Input: part model. Units: mm. Frame: model coordinates. Face numbers are marked on the shaded views. A direction names the side the tool comes from. Coordinates: 2 decimals unless noted, no trailing zeros. Write each loop counter-clockwise with the first axis right and the second up, starting at its lowest first coordinate (ties: lowest second). Pieces come first, ordered by that corner, then holes. Notation, with made-up numbers: (-20.5, 35) -> (-8.5, 35) arc R16 cw to (-8.5, 51) -> close; hole circle Ø11 at (-17.75, 41). An arc over 180 degrees is marked (long way). One line per question, with ' | ' between items. Start each with the question number.
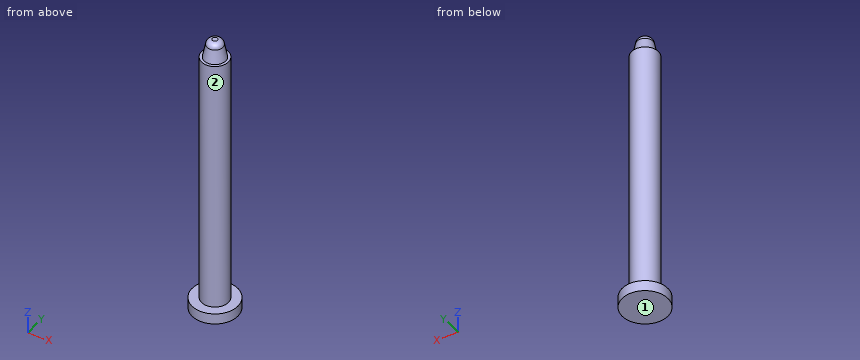
```python
from build123d import *

# Parameters (mm, degrees)
F0_R     = 8.5
F1_DEPTH = 4
F2_R     = 5
F3_DEPTH = 100


with BuildPart() as f1:
    # F0 (on Top) → F1 (new body)
    with BuildSketch(Plane.XY):
        Circle(F0_R)
    extrude(amount=F1_DEPTH)

    # F2 (on Top) → F3 (join)
    with BuildSketch(Plane.XY):
        Circle(F2_R)
    extrude(amount=F3_DEPTH)

    # F4 (on Right) → F5 (revolve)
    with BuildSketch(Plane.YZ):
        Polygon((3, 105), (0, 105), (0, 100), (4, 100), align=None)
    revolve(axis=Axis((0, 0, 102.5), (0, 0, -1)))

    # F6 (on Right) → F7 (revolve)
    with BuildSketch(Plane.YZ):
        with BuildLine():
            Line((1, 107), (0, 107))
            Line((0, 107), (0, 105))
            Line((0, 105), (3, 105))
            ThreePointArc((3, 105), (2.414214, 106.414214), (1, 107))
        make_face()
    revolve(axis=Axis((0, 0, 106), (0, 0, -1)))


solid = f1.part
```
1) Section B-B, the plane y = 7.5. Return loops of the section in (x, z).
2) First-contact query: P1, Ø3, axis at y = 4.5, z = 43.5, coming from the -X side; P2, Ø1.5, axis at y = -1.5, z = 26.5, coming from the -X side; P3, Ø8, axis at y = -5, z = 15, coming from the +X side. Flat tips, straight axial feed; report the tip coordinate or a pass-through.
3) Access query for the marked faces 1 and 2. Directions: +Z, -Z, +X, -X, +Y, -Y. A direction counts if a zero-diameter tool reaches every point of the face in a straight line with its end or side. Return the directions, or none.
4) Section C-C, the plane x = -6.25. Return loops of the section in (y, z).
5) Section A-A, the plane z = 22.5. Return loops of the section in (x, y), then the cut area to 3 significant figures.
6) Ray query, line 1 (Y direction, x = -3, z = 26.5); line 2 (Z direction, x = 7, y = 3.75); line 3 (Z direction, x = -1.25, y = 4). Return the intervals inside material, ascending.
Answer block:
1) outline: (-4, 0) -> (4, 0) -> (4, 4) -> (-4, 4) -> close
2) P1: stops at x = -4 | P2: stops at x = -4.94 | P3: stops at x = 4.9
3) face 1: -Z, +X, -X, +Y, -Y | face 2: +Z
4) outline: (-5.76, 0) -> (5.76, 0) -> (5.76, 4) -> (-5.76, 4) -> close
5) outline: circle Ø10 at (0, 0) | area: 78.5 mm2
6) line 1: y = -4 to 4 | line 2: z = 0 to 4 | line 3: z = 0 to 100
